CAD build for the part. Positions are in the model's coordinates, mm. A direction names the side the tool comes from. Give positions to 0.01 mm unless a question says otherwise; leave off trailing zeros. Loops run counter-clockwise (first coordinate to the right, second up) from the corner with the lowest first, then second, coordinate; pieces in that order, holes last. Notation, with made-up numbers: M -10.5,-11 L 31.5,-11 A28 cw 31.5,17 Z; hole C 48.5,8 d11. An arc over 180 degrees is marked long. One line per question, with ' | ' between items.
```python
from build123d import *

# Parameters (mm, degrees)
ESBO_O1_W                = 10
ESBO_O1_H                = 42
ESBO_O1_R                = 1.75
RESSALTO_EXTRUS_O1_DEPTH = 5
ESBO_O2_W                = 10
ESBO_O2_H                = 70
ESBO_O2_R                = 2
RESSALTO_EXTRUS_O2_DEPTH = 5


with BuildPart() as part:
    # Esboço1 → Ressalto-extrusão1 (new body)
    with BuildSketch(Plane.XY):
        Rectangle(ESBO_O1_W, ESBO_O1_H)
        with Locations((0, 15.5)):
            Circle(ESBO_O1_R, mode=Mode.SUBTRACT)
        with Locations((0, -15.5)):
            Circle(ESBO_O1_R, mode=Mode.SUBTRACT)
    extrude(amount=RESSALTO_EXTRUS_O1_DEPTH)

    # Esboço2 → Ressalto-extrusão2 (add)
    with BuildSketch(Plane.XZ.offset(21)):
        with Locations((0, -10)):
            Rectangle(ESBO_O2_W, ESBO_O2_H)
        with Locations(Location((0, 20, 0), (0, 0, 270))):
            Circle(ESBO_O2_R, mode=Mode.SUBTRACT)
        with Locations(Location((0, -40, 0), (0, 0, 270))):
            Circle(ESBO_O2_R, mode=Mode.SUBTRACT)
        with Locations(Location((0, 10, 0), (0, 0, 270))):
            Circle(ESBO_O2_R, mode=Mode.SUBTRACT)
    extrude(amount=RESSALTO_EXTRUS_O2_DEPTH)


solid = part.part
```
Item 1: Saw through at B-B on y = -15.5. Give the cut face in (x, z), and give its area (3 significant figures).
Conclusion:
outline: M -5,0 L -1.75,0 L -1.75,5 L -5,5 Z; M 1.75,0 L 5,0 L 5,5 L 1.75,5 Z | area: 32.5 mm²
Item 2: Saw through at A-A on z = -40. Give the cut face in (x, y), and give its area (3 significant figures).
Conclusion:
outline: M -5,-26 L -2,-26 L -2,-21 L -5,-21 Z; M 2,-26 L 5,-26 L 5,-21 L 2,-21 Z | area: 30.0 mm²
Item 3: 3-axis set-ups, long thin cutter, end or side, ignore diameter. For faces 1 (the cylindrical face through (-0.228, -13.765, 2.465)), 2 (the flat face through (0, -21, 15)), 3 (the flat face through (0, 0, 0)): which of +Z, -Z, +X, -X, +Y, -Y reach the whole face in a straight line?
Conclusion:
face 1: +Z, -Z | face 2: +Z, +X, -X, +Y | face 3: -Z, +X, -X, +Y
Item 4: Mould opens along Z. For faces 4 (the flat face through (0, 21, 2)), 5 (the cylindrical face through (-1.2, -23.5, 11.6)), 6 (the flat face through (0, 0, 5)) say: pulls with the +Z half, pulls with the -Z half, needs draft (parallel to the pull), parting line crosses it, or undercut.
Conclusion:
face 4: needs draft | face 5: undercut | face 6: pulls with the +Z half
Item 5: Drop flat-ended pins along their axis: P1, Ø5, axis at x = 1, y = 4, coming from the +Z side; P2, Ø2, axis at x = 1.5, z = -11.5, coming from the +Y side. Give the stop position or say it passes through.
Conclusion:
P1: z = 5 | P2: y = -21
Item 6: Saw through at D-D on y = -22.5. Give the cut face in (x, z), and give its area (3 significant figures).
Conclusion:
outline: M -5,-45 L 5,-45 L 5,25 L -5,25 Z; hole C 0,-40 d4; hole C 0,10 d4; hole C 0,20 d4 | area: 662 mm²
Item 7: Saw through at C-C on x = -1. Give the cut face in (y, z).
Conclusion:
outline: M -26,-45 L -21,-45 L -21,-41.73 L -26,-41.73 Z; M -26,-38.27 L -21,-38.27 L -21,0 L -16.94,0 L -16.94,5 L -21,5 L -21,8.27 L -26,8.27 Z; M -26,11.73 L -21,11.73 L -21,18.27 L -26,18.27 Z; M -26,21.73 L -21,21.73 L -21,25 L -26,25 Z; M -14.06,0 L 14.06,0 L 14.06,5 L -14.06,5 Z; M 16.94,0 L 21,0 L 21,5 L 16.94,5 Z
Item 8: Drill centre lines: line 1 along X through (y, z) = (-23.2, 20); line 2 along Z through (x, y) = (-1.25, -22); line 3 along Y through (x, z) = (0.25, 4). Where is each one in solid material? Low to high. Write a range as [from, to].
Conclusion:
line 1: [-5, -2], [2, 5] | line 2: [-45, -41.56], [-38.44, 8.44], [11.56, 18.44], [21.56, 25] | line 3: [-26, -17.23], [-13.77, 13.77], [17.23, 21]
